Drawing for the job (mm, zero at the part's lowest x, y, z). A direction names the side the tool comes from. Round coordinates to 2 decimals unless told otherwise and drop trailing zeros. Order: outer loops, then holes, each group sorted by start corner. A loop starts at its lowest first (then second) coordinate and runs counter-clockwise, first axis right, second up. Notation, with made-up numbers: (7, 33) - (54, 33) arc R35 ccw to (54, 70) - close; hole circle Ø6 at (14, -29). An arc over 180 degrees is marked (long way). Answer as a JSON object with one key per item and string values.
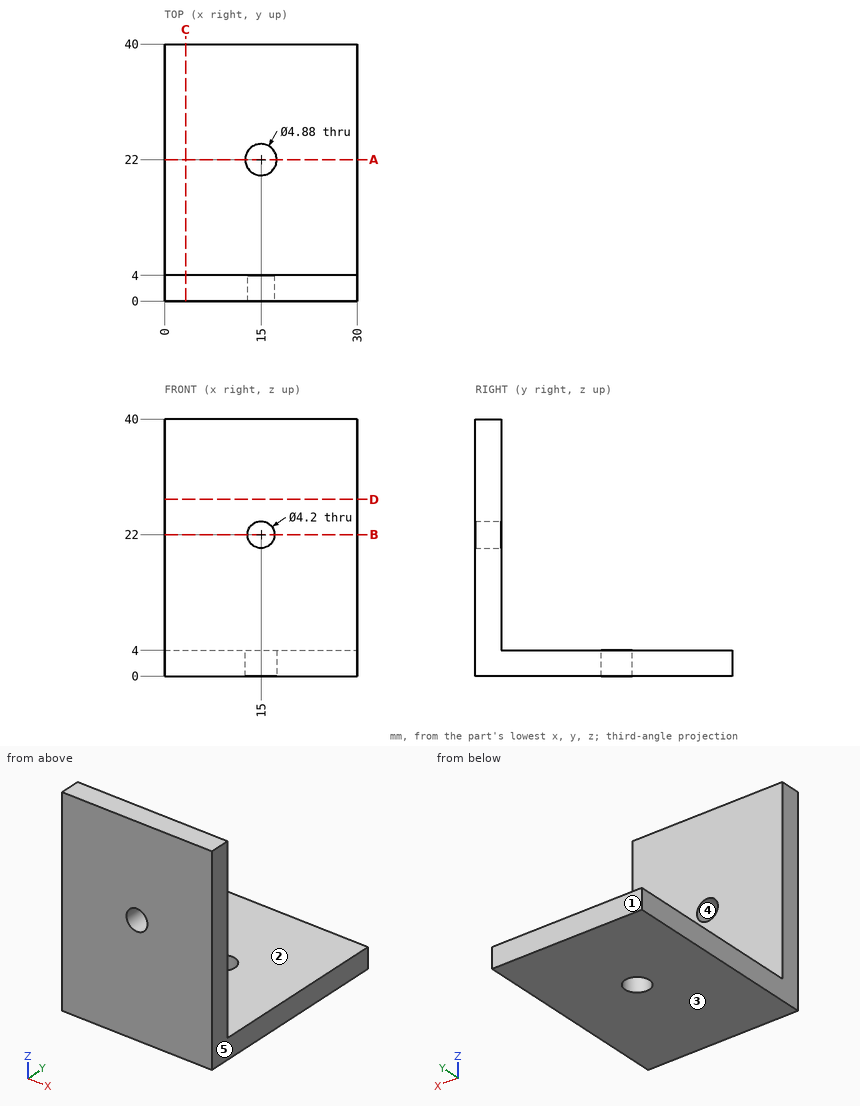
Item 1: Tool access for the marked faces 1 and 2: list every direction of +Z, -Z, +X, -X, +Y, -Y with a clear straight run to the whole face (end or side of a thin tool).
Taken from the geometry:
{"face 1": "+Z, -Z, +X, -X, +Y", "face 2": "+Z, +X, -X, +Y"}
Item 2: Drop flat-ended pins along their axis: P1, Ø8, axis at x = 15, y = 22, coming from the +Z side; P2, Ø15, axis at x = 21.5, z = 25.5, coming from the +Y side. Give the stop position or say it passes through.
Taken from the geometry:
{"P1": "z = 4", "P2": "y = 4"}
Item 3: Probe L1, parallel to Z at x = 15, y = 2.25; L2, parallel to Y at x = 2, z = 31.5. List the from-to ranges inside material, lowest first. Write a range as from..to.
Taken from the geometry:
{"L1": "0..19.9, 24.1..40", "L2": "0..4"}
Item 4: Cut at C-C (x = 3.25). Write the cut outline in (y, z), plus the area to 3 significant figures.
Taken from the geometry:
{"outline": "(0, 0) - (40, 0) - (40, 4) - (4, 4) - (4, 40) - (0, 40) - close", "area": "304 mm2"}
Item 5: Cut at D-D (z = 27.5). Write the cut outline in (x, y).
Taken from the geometry:
{"outline": "(0, 0) - (30, 0) - (30, 4) - (0, 4) - close"}
Item 6: Cut at A-A (y = 22). Write the cut outline in (x, z).
Taken from the geometry:
{"outline": "(0, 0) - (12.56, 0) - (12.56, 4) - (0, 4) - close; (17.44, 0) - (30, 0) - (30, 4) - (17.44, 4) - close"}
Item 7: Two-plate mould, pull along X, no slides. Class the marked faces 3, 4 and 5: pulls with the +X half, pulls with the -X half, needs draft (parallel to the pull), parting line crosses it, or undercut.
Taken from the geometry:
{"face 3": "needs draft", "face 4": "undercut", "face 5": "pulls with the +X half"}
Item 8: Cut at B-B (z = 22). Write the cut outline in (x, y).
Taken from the geometry:
{"outline": "(0, 0) - (12.9, 0) - (12.9, 4) - (0, 4) - close; (17.1, 0) - (30, 0) - (30, 4) - (17.1, 4) - close"}
